```python
from build123d import *

# Parameters (mm, degrees)
F1_DEPTH = 40
F2_W     = 60
F2_H     = 15
F3_DEPTH = 55
F5_DEPTH = 38.1
F6_R     = 10
F7_DEPTH = 25.4
F8_R     = 5
F9_DEPTH = 25.4


with BuildPart() as f1:
    # F0 (on Front) → F1 (new body)
    with BuildSketch(Plane.XZ):
        Polygon((-30, 20), (-30, 0), (-20, 0), (-20, 10), (20, 10), (20, 0), (30, 0), (30, 20), align=None)
    extrude(amount=F1_DEPTH)

    # F2 (on face) → F3 (join)
    with BuildSketch(Plane.XY.offset(20)):
        with Locations((0, -7.5)):
            Rectangle(F2_W, F2_H)
    extrude(amount=F3_DEPTH)

    # F4 (on face) → F5 (cut)
    with BuildSketch(Plane.XZ.offset(15)):
        Polygon((-30, 60), (-15, 75), (-30, 75), align=None)
    extrude(amount=-F5_DEPTH, mode=Mode.SUBTRACT)

    # F6 (on face) → F7 (cut)
    with BuildSketch(Plane.XZ.offset(15)):
        with Locations((0, 40)):
            Circle(F6_R)
    extrude(amount=-F7_DEPTH, mode=Mode.SUBTRACT)

    # F8 (on face) → F9 (cut)
    with BuildSketch(Plane.XY.offset(20)):
        with Locations((0, -27.5)):
            Circle(F8_R)
    extrude(amount=-F9_DEPTH, mode=Mode.SUBTRACT)


solid = f1.part
```
Can you work these out from the model? Positions are in its coordinate system, mm. A direction names the side the tool comes from. Coordinates: 2 decimals unless noted, no trailing zeros. Loops run counter-clockwise (first coordinate to the right, second up) from the corner with the lowest first, then second, coordinate; pieces in that order, holes last.
1) Imagine slicing it at D-D on x = 6. List the corners of the cut face in (y, z) for me, plus the area to 3 significant figures.
2) For pin 1 (8 mm diameter, centred on x = 16.5, y = -28.5, fed in from +Z); pin 2 (5 mm diameter, centred on y = -15.5, z = 43, fed in from +X); pin 3 (16.5 mm diameter, centred on x = -6.5, z = 51.5, fed in from -Y); pin 4 (8 mm diameter, centred on x = 0, y = -27.5, fed in from -Z), each with a flat end and sliding along its axis, tell me the tip position at first contact or that it passes through.
3) Which directions (+Z, -Z, +X, -X, +Y, -Y) give clear straight access to the entire face, cutting with the end or side of a thin tool? Please do faces 5 (the flat face through (0, -22, 20)), 6 (the flat face through (20, -20, 5)), 7 (the flat face through (30, -11, 29)).
4) I need wall thicknesses on probe 1 along Z at (x, y) = (0, -12); probe 2 along Y at (x, z) = (0, 16); probe 3 along X at (y, z) = (-4, 8). Which ranges of each line are inside material? Lowest first, please.
5) Imagine slicing it at B-B on x = 0. List the corners of the cut face in (y, z) for me, plus the area to 3 significant figures.
6) Imagine slicing it at C-C on y = -27.5. List the corners of the cut face in (x, z) for me.
7) Imagine slicing it at A-A on z = 40. List the corners of the cut face in (x, y) for me, plus the area to 3 significant figures.
8) Thinking about a two-plate mould opening in X: for faces 1 (the cylindrical face through (-2.17, -7.6, 30.24)), 2 (the flat face through (-20, -20, 5)), 3 (the flat face through (0, -15, 53)), 4 (the flat face through (-30, -11, 23)), which applies, pulls with the +X half, pulls with the -X half, needs draft (parallel to the pull), parting line crosses it, or undercut?
Completed:
1. outline: (-40, 10) - (0, 10) - (0, 32) - (-15, 32) - (-15, 20) - (-40, 20) - close; (-15, 48) - (0, 48) - (0, 75) - (-15, 75) - close
1. area: 985 mm2
2. pin 1: stops at z = 20
2. pin 2: stops at x = 30
2. pin 3: stops at y = -15
2. pin 4: passes through
3. face 5: +Z, +X, -X, -Y
3. face 6: -Z, +Y, -Y
3. face 7: +Z, -Z, +X, +Y, -Y
4. probe 1: z = 10 to 30, 50 to 75
4. probe 2: y = -40 to -32.5, -22.5 to 0
4. probe 3: x = -30 to -20, 20 to 30
5. outline: (-40, 10) - (-32.5, 10) - (-32.5, 20) - (-40, 20) - close; (-22.5, 10) - (0, 10) - (0, 30) - (-15, 30) - (-15, 20) - (-22.5, 20) - close; (-15, 50) - (0, 50) - (0, 75) - (-15, 75) - close
5. area: 825 mm2
6. outline: (-30, 0) - (-20, 0) - (-20, 10) - (-5, 10) - (-5, 20) - (-30, 20) - close; (5, 10) - (20, 10) - (20, 0) - (30, 0) - (30, 20) - (5, 20) - close
7. outline: (-30, -15) - (-10, -15) - (-10, 0) - (-30, 0) - close; (10, -15) - (30, -15) - (30, 0) - (10, 0) - close
7. area: 600 mm2
8. face 1: undercut
8. face 2: undercut
8. face 3: needs draft
8. face 4: pulls with the -X half
